```python
from build123d import *

# Parameters (mm, degrees)
EXTRUDE_1_DEPTH = 4


with BuildPart() as part:
    # Эскиз1 → Бобышка-Вытянуть1 (new body)
    with BuildSketch(Plane(origin=(0, 0, 0), x_dir=(1, 0, 0), z_dir=(0, 1, 0))):
        Polygon((0, 0), (0, -9), (9.093856713, -9), (16, -5.779612497), (16, 0), align=None)
    extrude(amount=EXTRUDE_1_DEPTH)

    # Эскиз2 → Цековка для  винта с внутренним шестигранником #41 (revolve, cut)
    with BuildSketch(Plane(origin=(10.5, 4, 4.5), x_dir=(0, 0, 1), z_dir=(1, 0, 0))):
        Polygon((0, 0), (0, 4), (1.6002, 4), (1.4732, 3.873), (1.4732, 2.9718), (1.6002, 2.8448), (2.77876, 2.8448), (2.77876, 0), align=None)
    revolve(axis=Axis((10.5, 10.35, 4.5), (0, -1, 0)), mode=Mode.SUBTRACT)


solid = part.part
```
Geometry: final body of the model. Coordinates: model frame, mm. A direction names the side the tool comes from. Round coordinates to 2 decimals unless told otherwise and drop trailing zeros. Loops run counter-clockwise (first coordinate to the right, second up) from the corner with the lowest first, then second, coordinate; pieces in that order, holes last.
Item 1: Line query: L1, parallel to X at y = 2.05, z = 4.5; L2, parallel to Z at x = 9.25, y = 2.35; L3, parallel to Y at x = 8.5, z = 4. Output: solid intervals per line, ascending.
Checked values:
L1: x = 0 to 7.72, 13.28 to 16
L2: z = 0 to 2.02, 6.98 to 8.93
L3: y = 0 to 1.16
Item 2: Section B-B, the plane y = 2.4. Output: boundary loops of the cut face in (x, z).
Checked values:
outline: (0, 0) - (16, 0) - (16, 5.78) - (9.09, 9) - (0, 9) - close; hole circle Ø5.56 at (10.5, 4.5)
Item 3: Section C-C, the plane x = 10.5. Output: boundary loops of the cut face in (y, z).
Checked values:
outline: (0, 0) - (4, 0) - (4, 1.72) - (1.16, 1.72) - (1.16, 2.9) - (1.03, 3.03) - (0.13, 3.03) - (0, 2.9) - close; (0, 6.1) - (0.13, 5.97) - (1.03, 5.97) - (1.16, 6.1) - (1.16, 7.28) - (4, 7.28) - (4, 8.34) - (0, 8.34) - close
Item 4: Mould query, pull axis Z, two halves, no side actions, for faces 3 (the flat face through (8, 2, 0)), 4 (the flat face through (12, 1.155, 3)), 5 (the flat face through (4, 2, 9)). Classes: released by +Z, released by -Z, zero draft, split by the parting line, or undercut.
Checked values:
face 3: released by -Z
face 4: undercut
face 5: released by +Z
Item 5: Section D-D, the plane z = 6.5. Output: boundary loops of the cut face in (x, y).
Checked values:
outline: (0, 0) - (14.46, 0) - (14.46, 4) - (12.43, 4) - (12.43, 1.16) - (8.57, 1.16) - (8.57, 4) - (0, 4) - close
Item 6: Contact query for a flat-ended pin moving along its axis: P1, Ø1.7, axis at x = 9.5, z = 6, coming from the +Y side. Output: stop coordinate, or through.
Checked values:
P1: stops at y = 1.16
Item 7: Reachability of faces 1 (the flat face through (6, 4, 4)), 2 (the cylindrical face through (8.622, 2.598, 2.452)) from +Z, -Z, +X, -X, +Y, -Y: full face, straight path, thin tool, end or side. Return the list, or none.
Checked values:
face 1: +Z, -Z, +X, -X, +Y
face 2: +Y
Item 8: Section A-A, the plane z = 4.5. Output: boundary loops of the cut face in (x, y).
Checked values:
outline: (0, 0) - (8.9, 0) - (9.03, 0.13) - (9.03, 1.03) - (8.9, 1.16) - (7.72, 1.16) - (7.72, 4) - (0, 4) - close; (11.97, 0.13) - (12.1, 0) - (16, 0) - (16, 4) - (13.28, 4) - (13.28, 1.16) - (12.1, 1.16) - (11.97, 1.03) - close
